Source: CAD feature listing. Evaluate the final solid. Frame: model axes, mm. A direction names the side the tool comes from. Coordinates: 2 decimals unless noted, no trailing zeros. Order: outer loops, then holes, each group sorted by start corner. A loop starts at its lowest first (then second) coordinate and runs counter-clockwise, first axis right, second up.
```python
from build123d import *

# Parameters (mm, degrees)
F0_W     = 94.539702
F0_H     = 57.64192
F1_DEPTH = 25.4
F2_T     = -2.54
F4_D     = 3.81


with BuildPart() as f1:
    # F0 (on Top) → F1 (new body)
    with BuildSketch(Plane.XY):
        Rectangle(F0_W, F0_H)
    extrude(amount=F1_DEPTH)

    # F2
    f2_openings = [f1.faces().sort_by_distance(p)[0] for p in [
        (0, 0, 25.4),
        (0, -28.82096, 12.7),
    ]]
    offset(amount=F2_T, openings=f2_openings)

    # F4 (through all)
    with Locations(Plane.XZ.offset(-26.28096)):
        with Locations((0, 12.345429)):
            Hole(F4_D / 2)


solid = f1.part
```
1. Pin query (flat end, axial travel): P1, Ø1.5, axis at x = 0.5, y = -21, coming from the +Z side; P2, Ø8, axis at x = 3.5, z = 11.5, coming from the -Y side; P3, Ø6, axis at x = 0, z = 12.35, coming from the +Y side. Return the tip coordinate at first contact, or that it passes through.
Findings:
P1: stops at z = 2.54
P2: stops at y = 26.28
P3: stops at y = 28.82
2. Access query for faces 4 (the face through (0, 28, 25.4)), 5 (the face through (-1, 26.281, 16)). Directions: +Z, -Z, +X, -X, +Y, -Y. A direction counts if a zero-diameter tool reaches every point of the face in a straight line with its end or side. Return the directions, or none.
Findings:
face 4: +Z, +X, -X, +Y, -Y
face 5: +Z, -Y
3. Section query D-D on x = -39.5. Return loops of the section in (y, z), plus the area to 3 significant figures.
Findings:
outline: (-28.82, 0) - (28.82, 0) - (28.82, 25.4) - (26.28, 25.4) - (26.28, 2.54) - (-28.82, 2.54) - close
area: 204 mm2
4. Section query C-C on y = 5. Return loops of the section in (x, z).
Findings:
outline: (-47.27, 0) - (47.27, 0) - (47.27, 25.4) - (44.73, 25.4) - (44.73, 2.54) - (-44.73, 2.54) - (-44.73, 25.4) - (-47.27, 25.4) - close
5. Section query A-A on x = 0. Return loops of the section in (y, z).
Findings:
outline: (-28.82, 0) - (28.82, 0) - (28.82, 10.44) - (26.28, 10.44) - (26.28, 2.54) - (-28.82, 2.54) - close; (26.28, 14.25) - (28.82, 14.25) - (28.82, 25.4) - (26.28, 25.4) - close
6. Draft query along X for faces 1 (the face through (0, -28.821, 2)), 2 (the face through (-47.27, 0, 13)), 3 (the face through (-1, -1, 2.54)). Return one class per face: released by +X, released by -X, zero draft, split by the parting line, or undercut.
Findings:
face 1: zero draft
face 2: released by -X
face 3: undercut
7. Section query B-B on z = 17.75. Return loops of the section in (x, y).
Findings:
outline: (-47.27, -28.82) - (-44.73, -28.82) - (-44.73, 26.28) - (44.73, 26.28) - (44.73, -28.82) - (47.27, -28.82) - (47.27, 28.82) - (-47.27, 28.82) - close
8. Ray query, line 1 (X direction, y = 8, z = 22.25); line 2 (Z direction, x = 0, y = 27.25); line 3 (Y direction, x = -11, z = 14.5). Return the intervals inside material, ascending.
Findings:
line 1: x = -47.27 to -44.73, 44.73 to 47.27
line 2: z = 0 to 10.44, 14.25 to 25.4
line 3: y = 26.28 to 28.82
